Input: dimensioned drawing with shaded views. Units: mm. Origin: part minimum x, y, z. Give positions to 0.01 mm unless a question says otherwise; leave off trailing zeros. Order: outer loops, then holes, each group sorted by start corner. A loop starts at its lowest first (then second) coordinate and runs counter-clockwise, first axis right, second up. Notation, with made-up numbers: (24.25, -4.75) -> (52.25, -4.75) arc R19 cw to (52.25, 32.25) -> close; hole circle Ø8 at (14.5, 67). An arc over 180 degrees is marked (long way). One line per question, with ' | ' between items. Start each with the question number.
(1) First-contact query: pin 1 Ø8 at (y, z) = (87, 30) entering from +X; pin 2 Ø2 at (x, y) = (19.5, 46) entering from +Z (1 decimal); pin 3 Ø4 at (x, y) = (61.5, 54) entering from -Z. Flat tips, straight axial feed; report the tip coordinate or a pass-through.
(2) Section C-C (z = 28.5). Return loops of the section in (x, y).
(3) Section A-A (y = 58.5). Return loops of the section in (x, z) (1 decimal).
(4) Section B-B (x = 17). Return loops of the section in (y, z), then the cut area to 3 significant figures.
(5) Ray query, L1, parallel to X at y = 80.5, z = 58.5 (1 decimal); L2, parallel to X at y = 23, z = 58 (1 decimal); L3, parallel to Z at x = 24.5, y = 66 (1 decimal). Return the intervals inside material, ascending.
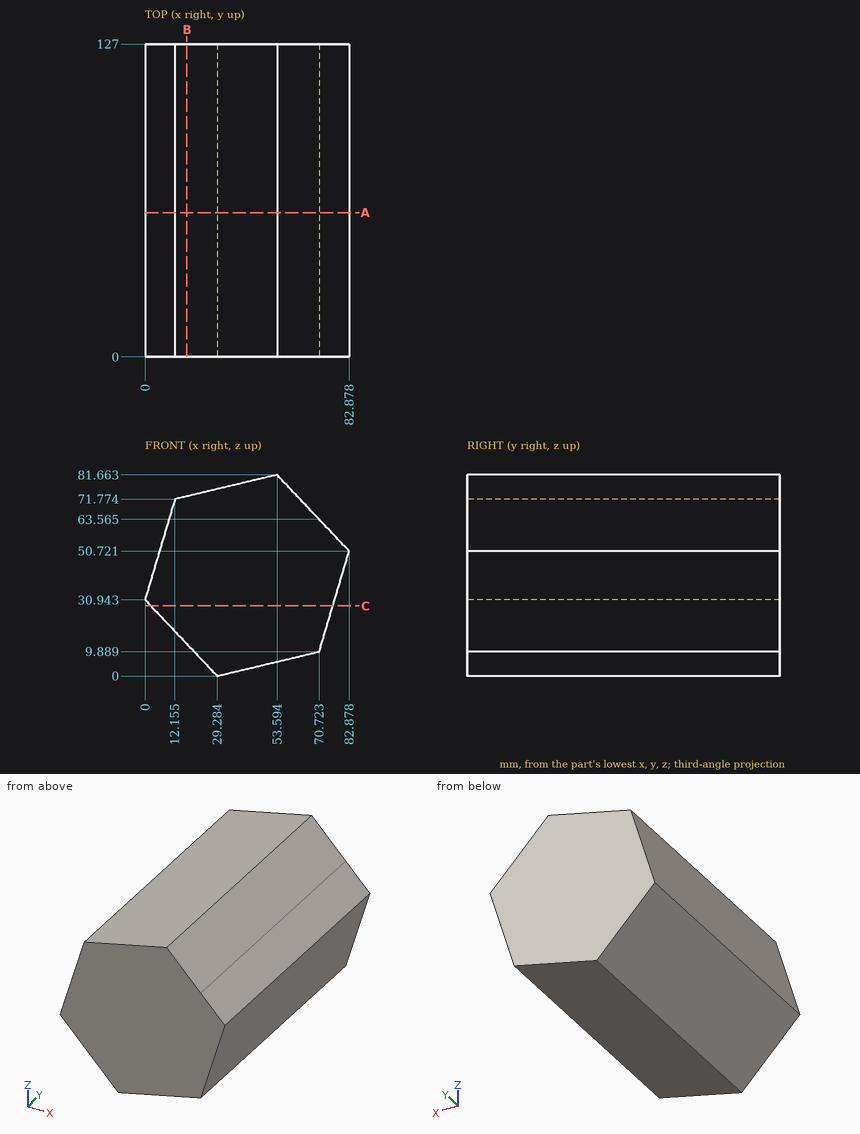
Response:
1) pin 1: stops at x = 77.9 | pin 2: stops at z = 73.8 | pin 3: stops at z = 7.21
2) outline: (2.31, 0) -> (76.26, 0) -> (76.26, 127) -> (2.31, 127) -> close
3) outline: (0, 30.9) -> (29.3, 0) -> (70.7, 9.9) -> (82.9, 50.7) -> (53.6, 81.7) -> (12.2, 71.8) -> close
4) outline: (0, 12.98) -> (127, 12.98) -> (127, 72.93) -> (0, 72.93) -> close | area: 7,610 mm^2
5) L1: x = 8.2 to 75.5 | L2: x = 8.1 to 76 | L3: z = 5.1 to 74.7
